Could you check a few things on this drawing? It's one solid part, dimensions in mm from its lowest x, y, z. A direction names the side the tool comes from. Coordinates: 2 decimals unless noted, no trailing zeros. Loops run counter-clockwise (first coordinate to the right, second up) from the corner with the lowest first, then second, coordinate; pieces in that order, holes last. Notation, with made-up numbers: (42, -4) -> (58, -4) arc R12 cw to (58, 4) -> close; hole circle Ø8 at (-32.75, 10.25). An arc over 180 degrees is marked (long way). One line per question, with ' | ' between items.
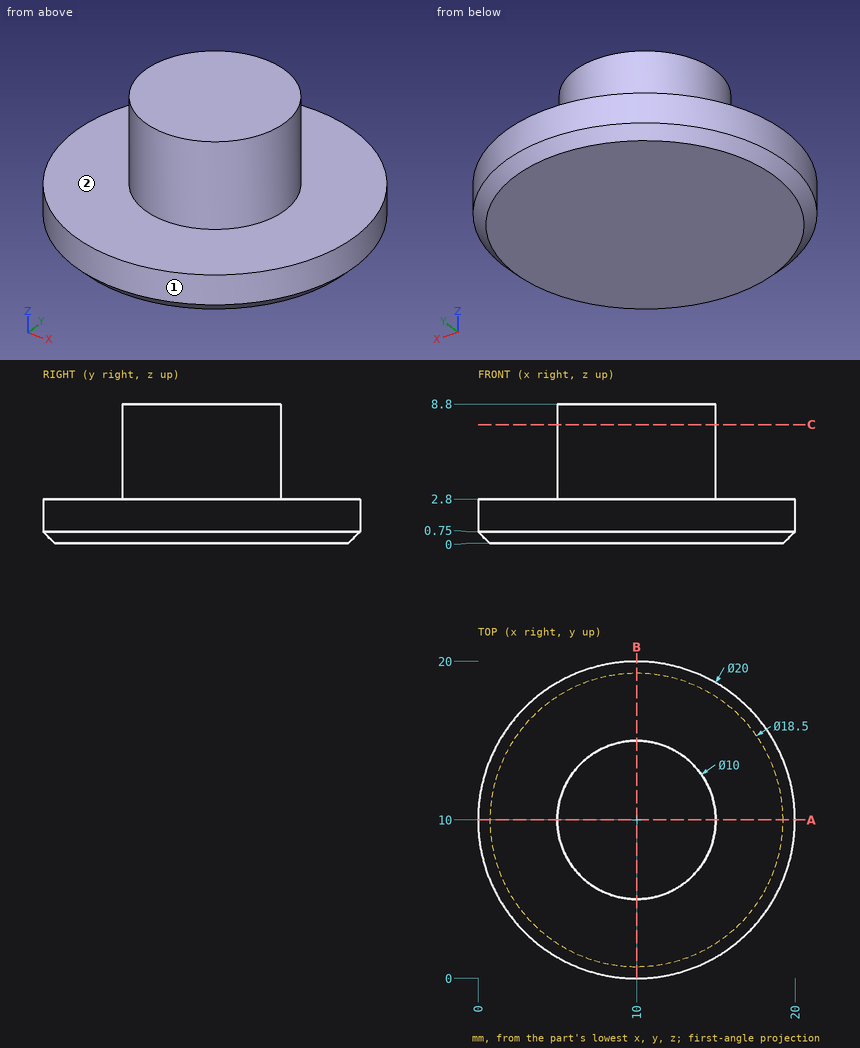
1) I need wall thicknesses on line 1 along Z through (x, y) = (1, 10.25); line 2 along Y through (x, z) = (8.75, 2); line 3 along Z through (x, y) = (16, 2.25). Which ranges of each line are inside material? Lowest first, please. Write a range as from..to.
Data:
line 1: 0..2.8 | line 2: 0.08..19.92 | line 3: 0.55..2.8
2) I'm going to push flat-ended pins straight in: pin 1 Ø3 at (y, z) = (7.5, 5.5) entering from -X; pin 2 Ø4 at (x, y) = (4, 17) entering from +Z; pin 3 Ø1.5 at (x, z) = (16.5, 6) entering from +Y; pin 4 Ø3 at (y, z) = (8, 2.5) entering from -X. Where does each tip first touch, or does it pass through?
Data:
pin 1: x = 5.1 | pin 2: z = 2.8 | pin 3: through | pin 4: x = 0.01
3) If we section it at C-C on z = 7.5: Please give me the cut outline in (x, y).
Data:
outline: circle Ø10 at (10, 10)
4) On a 3-axis mill with a long thin cutter (end or side, diameter ignored), from which of +Z, -Z, +X, -X, +Y, -Y can I reach the whole of each face in a straight line? I mean the marked faces 1 and 2. Say none if no direction works.
Data:
face 1: +Z, -Z | face 2: +Z
5) If we section it at A-A on y = 10: Please give me the cut outline in (x, z).
Data:
outline: (0, 0.75) -> (0.75, 0) -> (19.25, 0) -> (20, 0.75) -> (20, 2.8) -> (15, 2.8) -> (15, 8.8) -> (5, 8.8) -> (5, 2.8) -> (0, 2.8) -> close
